```python
from build123d import *

# Parameters (mm, degrees)
SKETCH1_W                   = 1930.4
SKETCH1_H                   = 203.2
BOSS_EXTRUDE1_DEPTH         = 12.7
CUT_EXTRUDE1_DEPTH          = 13.7
FILLET1_R                   = 3.175
F_1_4_0_25_DIAMETER_HOLE1_D = 6.35


with BuildPart() as part:
    # Sketch1 → Boss-Extrude1 (new body)
    with BuildSketch(Plane(origin=(0, 0, 0), x_dir=(1, 0, 0), z_dir=(0, 1, 0))):
        Rectangle(SKETCH1_W, SKETCH1_H)
    extrude(amount=BOSS_EXTRUDE1_DEPTH)

    # Sketch2 → Cut-Extrude1 (cut, through all)
    with BuildSketch(Plane(origin=(0, 12.7, 0), x_dir=(1, 0, 0), z_dir=(0, 1, 0))):
        with BuildLine():
            Line((-876.3, 0), (-876.3, -101.6))
            Line((-876.3, -101.6), (-749.3, -101.6))
            Line((-749.3, -101.6), (-749.3, 0))
            ThreePointArc((-749.3, 0), (-812.8, 63.5), (-876.3, 0))
        make_face()
        with BuildLine():
            Line((-673.1, 0), (-673.1, -101.6))
            Line((-673.1, -101.6), (-546.1, -101.6))
            Line((-546.1, -101.6), (-546.1, 0))
            ThreePointArc((-546.1, 0), (-609.6, 63.5), (-673.1, 0))
        make_face()
        with BuildLine():
            Line((-469.9, 0), (-469.9, -101.6))
            Line((-469.9, -101.6), (-342.9, -101.6))
            Line((-342.9, -101.6), (-342.9, 0))
            ThreePointArc((-342.9, 0), (-406.4, 63.5), (-469.9, 0))
        make_face()
        with BuildLine():
            Line((-266.7, 0), (-266.7, -101.6))
            Line((-266.7, -101.6), (-139.7, -101.6))
            Line((-139.7, -101.6), (-139.7, 0))
            ThreePointArc((-139.7, 0), (-203.2, 63.5), (-266.7, 0))
        make_face()
        with BuildLine():
            Line((-63.5, 0), (-63.5, -101.6))
            Line((-63.5, -101.6), (63.5, -101.6))
            Line((63.5, -101.6), (63.5, 0))
            ThreePointArc((63.5, 0), (0, 63.5), (-63.5, 0))
        make_face()
        with BuildLine():
            Line((139.7, 0), (139.7, -101.6))
            Line((139.7, -101.6), (266.7, -101.6))
            Line((266.7, -101.6), (266.7, 0))
            ThreePointArc((266.7, 0), (203.2, 63.5), (139.7, 0))
        make_face()
        with BuildLine():
            Line((342.9, 0), (342.9, -101.6))
            Line((342.9, -101.6), (469.9, -101.6))
            Line((469.9, -101.6), (469.9, 0))
            ThreePointArc((469.9, 0), (406.4, 63.5), (342.9, 0))
        make_face()
        with BuildLine():
            Line((546.1, 0), (546.1, -101.6))
            Line((546.1, -101.6), (673.1, -101.6))
            Line((673.1, -101.6), (673.1, 0))
            ThreePointArc((673.1, 0), (609.6, 63.5), (546.1, 0))
        make_face()
        with BuildLine():
            Line((749.3, 0), (749.3, -101.6))
            Line((749.3, -101.6), (876.3, -101.6))
            Line((876.3, -101.6), (876.3, 0))
            ThreePointArc((876.3, 0), (812.8, 63.5), (749.3, 0))
        make_face()
    extrude(amount=-CUT_EXTRUDE1_DEPTH, mode=Mode.SUBTRACT)

    # Fillet1
    fillet1_edges = [part.edges().sort_by_distance(p)[0] for p in [
        (546.1, 6.35, 101.6),
        (876.3, 6.35, 101.6),
        (749.3, 6.35, 101.6),
        (-749.3, 6.35, 101.6),
        (-876.3, 6.35, 101.6),
        (-546.1, 6.35, 101.6),
        (-673.1, 6.35, 101.6),
        (-342.9, 6.35, 101.6),
        (-469.9, 6.35, 101.6),
        (-139.7, 6.35, 101.6),
        (-266.7, 6.35, 101.6),
        (-965.2, 6.35, 101.6),
        (-965.2, 6.35, -101.6),
        (965.2, 6.35, -101.6),
        (965.2, 6.35, 101.6),
        (63.5, 6.35, 101.6),
        (-63.5, 6.35, 101.6),
        (266.7, 6.35, 101.6),
        (139.7, 6.35, 101.6),
        (469.9, 6.35, 101.6),
        (342.9, 6.35, 101.6),
        (673.1, 6.35, 101.6),
    ]]
    fillet(fillet1_edges, radius=FILLET1_R)

    # 1/4 (0.25) Diameter Hole1 (through all)
    with Locations(Plane(origin=(0, 12.7, 0), x_dir=(1, 0, 0), z_dir=(0, 1, 0))):
        with Locations((-958.85, 76.2), (-958.85, 0), (-958.85, -76.2), (958.85, -76.2), (958.85, 0), (958.85, 76.2), (-914.4, -95.25), (-711.2, -95.25), (-508, -95.25), (-304.8, -95.25), (-101.6, -95.25), (101.6, -95.25), (304.8, -95.25), (508, -95.25), (711.2, -95.25), (914.4, -95.25)):
            Hole(F_1_4_0_25_DIAMETER_HOLE1_D / 2)


solid = part.part
```
Geometry check sheet. Reference: the model listing, model coordinates, mm. Round coordinates to 2 decimals unless told otherwise and drop trailing zeros. Order: outer loops, then holes, each group sorted by start corner. A loop starts at its lowest first (then second) coordinate and runs counter-clockwise, first axis right, second up. Notation, with made-up numbers: (-6, 59) -> (28, 59) arc R31 cw to (28, 86) -> close; hole circle Ø3 at (-17, 67.25). An arc over 180 degrees is marked (long way). Return JSON: item names as keys, results as strings. Group by question number.
Q1. Section check C-C, the plane x = 812.8. Record the boundary of the cut face in (y, z).
Q2. Section check A-A, the plane z = 19.5. Count the separate pieces of the cut face and the enclosed holes in it, plus the area to 4 significant figures.
Q3. Material ranges on probe 1 along Z at (x, y) = (-958.85, 8.25) (3 decimals); probe 2 along Z at (x, y) = (711.2, 8) (3 decimals); probe 3 along Z at (x, y) = (567.5, 4), recorded low to high. Write a range as from..to.
Q4. Section check D-D, the plane x = 237. Record the boundary of the cut face in (y, z).
Q5. Release check for a two-part mould opening along X. For faces 1 (the cylindrical face through (-811.404, 6.439, -63.485)), 2 (the flat face through (-5, 0, -83)) record: released by +X, released by -X, zero draft, split by the parting line, or undercut.
Numbers:
{
 "1": {"outline": "(0, -101.6) -> (12.7, -101.6) -> (12.7, -63.5) -> (0, -63.5) -> close"},
 "2": {"separate pieces": "10", "enclosed holes": "0", "area": "10,000 mm^2"},
 "3": {"probe 1": "-101.6..-79.375, -73.025..-3.175, 3.175..73.025, 79.375..101.6", "probe 2": "-101.6..92.075, 98.425..101.6", "probe 3": "-101.6..-47.54"},
 "4": {"outline": "(0, -101.6) -> (12.7, -101.6) -> (12.7, -53.76) -> (0, -53.76) -> close"},
 "5": {"face 1": "undercut", "face 2": "zero draft"}
}
